Check sheet for the modelled part. Datum: model origin and axes. Units: mm. A direction names the side the tool comes from. Give positions to 0.01 mm unless a question says otherwise; leave off trailing zeros. Write each loop counter-clockwise with the first axis right and the second up, starting at its lowest first coordinate (ties: lowest second). Pieces come first, ordered by that corner, then holes. Notation, with made-up numbers: (32, 17) -> (59, 17) arc R33 ccw to (59, 50) -> close; hole circle Ø2 at (19.5, 23.25). An arc over 180 degrees is marked (long way). Return JSON: item names as keys, results as strings.
Autodesk Inventor part; units mm, degrees
ref_plane "YZ Plane" through (0, 0, 0) normal (1, 0, 0) x (0, 1, 0)
ref_plane "XZ Plane" through (0, 0, 0) normal (0, 1, 0) x (-1, 0, 0)
ref_plane "XY Plane" through (0, 0, 0) normal (0, 0, 1) x (1, 0, 0)
sketch "Sketch1" plane through (0, 0, 0) normal (0, 1, 0) x (-1, 0, 0)
  line L0 (9.525, 0) -> (9.525, -28.8544)
  line L1 (9.525, -28.8544) -> (-9.525, -28.8544)
  line L2 (-9.525, -28.8544) -> (-9.525, 0)
  line L3 (-9.525, 0) -> (-12.7, 0)
  line L4 (-12.7, 0) -> (-12.7, -32.0294)
  line L5 (-12.7, -32.0294) -> (12.7, -32.0294)
  line L6 (12.7, -32.0294) -> (12.7, 0)
  line L7 (12.7, 0) -> (9.525, 0)
  line L8 (0, -38.4353) -> (0, 6.4059)
  line L9 (-17.78, 0) -> (17.78, 0)
  point P0 (0, 0)
  dimension "d0" = 3.175
  dimension "d1" = 19.05
  dimension "d2" = 28.8544
  dimension "d3" = 3.175
extrude "Extrusion1" add sketch "Sketch1" along normal mid plane 57.404 contours L7 L6 L5 L8 L1 L0 | L8 L5 L4 L3 L2 L1
sketch "Sketch2" plane through (12.7, 28.702, -32.0294) normal (0, 0, -1) x (-1, 0, 0)
  line L0 (25.4, -57.404) -> (25.4, 0)
  line L1 (0, 0) -> (25.4, 0)
  line L2 (0, -57.404) -> (0, 0)
  line L3 (25.4, -57.404) -> (0, -57.404)
  line L4 (12.7, -68.8848) -> (12.7, 11.4808)
  line L5 (-5.08, -28.702) -> (30.48, -28.702)
  circle A0 centre (12.7, -12.7) radius 3.175
  circle A1 centre (12.7, -44.704) radius 3.175
  point P0 (12.7, -28.702)
  dimension "d6" = 6.35
  dimension "d7" = 16.002
extrude "Extrusion2" cut sketch "Sketch2" against normal up to next contours A1 L4 | L4 A1 | A0 L4 | L4 A0
sketch "Sketch3" plane through (12.7, -28.702, -32.0294) normal (1, 0, 0) x (0, 0, -1)
  line L0 (0, 0) -> (0, 57.404)
  line L1 (-32.0294, 57.404) -> (0, 57.404)
  line L2 (-32.0294, 0) -> (-32.0294, 57.404)
  line L3 (0, 0) -> (-32.0294, 0)
  circle A0 centre (-19.3294, 14.4272) radius 3.175
  point P0 (-32.0294, 28.702)
  dimension "d10" = 6.35
  dimension "d11" = 12.7
  dimension "d12" = 14.4272
extrude "Extrusion3" cut sketch "Sketch3" against normal up to surface (25.4 mm away) contours A0
properties part number "Actuator Bracket"
(1) Cross-section at B-B on z = -22. Enter the section's corners in (x, y) (3 decimals), then the cut area to 3 significant figures.
Reply:
{"outline": "(-12.7, -28.702) -> (-9.525, -28.702) -> (-9.525, 28.702) -> (-12.7, 28.702) -> close; (9.525, -28.702) -> (12.7, -28.702) -> (12.7, 28.702) -> (9.525, 28.702) -> close", "area": "365 mm^2"}
(2) Set-up check for faces 1 (the flat face through (-9.525, 0, -14)), 2 (the flat face through (-11, 0, 0)): record each of +Z, -Z, +X, -X, +Y, -Y from which the full face is reachable in a straight line by a thin tool's end or side.
Reply:
{"face 1": "+Z, +Y, -Y", "face 2": "+Z, +X, -X, +Y, -Y"}
(3) Cross-section at A-A on x = 0. Enter the section's corners in (y, z), then the cut area to 3 significant figures.
Reply:
{"outline": "(-28.7, -32.03) -> (-19.18, -32.03) -> (-19.18, -28.85) -> (-28.7, -28.85) -> close; (-12.83, -32.03) -> (12.83, -32.03) -> (12.83, -28.85) -> (-12.83, -28.85) -> close; (19.18, -32.03) -> (28.7, -32.03) -> (28.7, -28.85) -> (19.18, -28.85) -> close", "area": "142 mm^2"}
(4) Cross-section at D-D on y = 14.5. Enter the section's corners in (x, z) (3 decimals).
Reply:
{"outline": "(-12.7, -32.029) -> (-2.797, -32.029) -> (-2.797, -28.854) -> (-9.525, -28.854) -> (-9.525, 0) -> (-12.7, 0) -> close; (2.797, -32.029) -> (12.7, -32.029) -> (12.7, 0) -> (9.525, 0) -> (9.525, -28.854) -> (2.797, -28.854) -> close"}
(5) Depth check by flat-ended pin: pin 1 Ø7.5 at (x, y) = (0, -16.002) entering from +Z; pin 2 Ø8 at (x, z) = (2, -20) entering from +Y. Enter the tip coordinate at first touch or a pass-through.
Reply:
{"pin 1": "z = -28.85", "pin 2": "through"}
(6) Release check for a two-part mould opening along Y. For faces 3 (the cylindrical face through (-3.03, -15.05, -30.46)), 4 (the flat face through (0, 0, -32.029)), 5 (the flat face through (-1, 28.702, -30)) record: pulls with the +Y half, pulls with the -Y half, needs draft (parallel to the pull), parting line crosses it, or undercut.
Reply:
{"face 3": "undercut", "face 4": "needs draft", "face 5": "pulls with the +Y half"}
(7) Cross-section at C-C on z = -12.7. Enter the section's corners in (x, y) (3 decimals).
Reply:
{"outline": "(-12.7, -28.702) -> (-9.525, -28.702) -> (-9.525, -17.45) -> (-12.7, -17.45) -> close; (-12.7, -11.1) -> (-9.525, -11.1) -> (-9.525, 28.702) -> (-12.7, 28.702) -> close; (9.525, -28.702) -> (12.7, -28.702) -> (12.7, -17.45) -> (9.525, -17.45) -> close; (9.525, -11.1) -> (12.7, -11.1) -> (12.7, 28.702) -> (9.525, 28.702) -> close"}
(8) Thickness scan on L1, parallel to Y at x = 0, z = -31.35; L2, parallel to X at y = 4, z = -7 (3 decimals); L3, parallel to Y at x = 11.2, z = -12.7. Record the ranges inside material, lowest first.
Reply:
{"L1": "-28.7 to -19.18, -12.83 to 12.83, 19.18 to 28.7", "L2": "-12.7 to -9.525, 9.525 to 12.7", "L3": "-28.7 to -17.45, -11.1 to 28.7"}
